from build123d import *

# Parameters (mm, degrees)
SKETCH1_W           = 56
SKETCH1_H           = 101
SKETCH1_R           = 1.65
BOSS_EXTRUDE1_DEPTH = 2
SKETCH3_W           = 56
SKETCH3_H           = 101
SKETCH3_W_2         = 50
SKETCH3_H_2         = 95
BOSS_EXTRUDE2_DEPTH = 15
SKETCH5_W           = 7
SKETCH5_H           = 72
CUT_EXTRUDE2_DEPTH  = 60.659450215


with BuildPart() as part:
    # Sketch1 → Boss-Extrude1 (new body)
    with BuildSketch(Plane(origin=(0, 0, 0), x_dir=(1, 0, 0), z_dir=(0, 1, 0))):
        Rectangle(SKETCH1_W, SKETCH1_H)
        with Locations(Location((-16.5, 40, 0), (0, 0, 270))):
            Circle(SKETCH1_R, mode=Mode.SUBTRACT)
        with Locations(Location((16.5, 40, 0), (0, 0, 270))):
            Circle(SKETCH1_R, mode=Mode.SUBTRACT)
        with Locations(Location((-16.5, -40, 0), (0, 0, 270))):
            Circle(SKETCH1_R, mode=Mode.SUBTRACT)
        with Locations(Location((16.5, -40, 0), (0, 0, 270))):
            Circle(SKETCH1_R, mode=Mode.SUBTRACT)
        Polygon((-12.964466094, -40), (12.964466094, -40), (16.5, -36.464466094), (16.5, 36.464466094), (12.964466094, 40), (-12.964466094, 40), (-16.5, 36.464466094), (-16.5, -36.464466094), align=None, mode=Mode.SUBTRACT)
    extrude(amount=BOSS_EXTRUDE1_DEPTH)

    # Sketch3 → Boss-Extrude2 (add)
    with BuildSketch(Plane(origin=(0, 2, 0), x_dir=(1, 0, 0), z_dir=(0, 1, 0))):
        Rectangle(SKETCH3_W, SKETCH3_H)
        Rectangle(SKETCH3_W_2, SKETCH3_H_2, mode=Mode.SUBTRACT)
    extrude(amount=BOSS_EXTRUDE2_DEPTH)

    # Sketch5 → Cut-Extrude2 (cut, through all)
    with BuildSketch(Plane(origin=(0, 2, 0), x_dir=(1, 0, 0), z_dir=(0, 1, 0))):
        with Locations((-20, 0)):
            Rectangle(SKETCH5_W, SKETCH5_H)
    extrude(amount=-CUT_EXTRUDE2_DEPTH, mode=Mode.SUBTRACT)


solid = part.part
Can you work these out from the model? Positions are in its coordinate system, mm. A direction names the side the tool comes from. Give positions to 0.01 mm unless a question says otherwise; leave off trailing zeros. Write each loop counter-clockwise with the first axis right and the second up, starting at its lowest first coordinate (ties: lowest second). Pieces come first, ordered by that corner, then holes. Notation, with made-up numbers: (-3.5, -37) -> (17.5, -37) arc R14 ccw to (17.5, -11) -> close; hole circle Ø11 at (79, 48.25). An arc over 180 degrees is marked (long way). Answer as a JSON object with one key per item and string values. Group by question number.
Item 1: Please list where these lines run through material, in increasing order: line 1 (Z direction, x = 11, y = 10.75); line 2 (X direction, y = 6.75, z = 18); line 3 (Y direction, x = -14.5, z = -40.5). Write a range as [from, to].
Item 2: For faces 4 (the face through (-20, 1, -36)), 5 (the face through (-25, 9, 1)), 6 (the face through (18, 0, -1)), which set-ups out of +Z, -Z, +X, -X, +Y, -Y let a thin tool reach every point of the face, with its end or its side?
Item 3: We'd pull the mould along X, two halves only. Please class faces 1 (the face through (-23.5, 1, 1)), 2 (the face through (28, 8, 1)), 3 (the face through (-27, 17, 4)): +X half, -X half, draft (parallel to the pull), parting line (faces both ways), or undercut.
Item 4: Suppose I cut it at C-C (y = 5.25). Please give me the cut outline in (x, z).
Item 5: Suppose I cut it at A-A (x = -8). Please give me the cut outline in (y, z), plus the area to 3 significant figures.
Item 6: Suppose I cut it at B-B (z = 9). Please give me the cut outline in (x, y), plus the area to 3 significant figures.
Item 7: Suppose I cut it at D-D (x = 24). Please give me the cut outline in (y, z), plus the area to 3 significant figures.
Findings:
{
 "1": {"line 1": "z = [-50.5, -47.5], [47.5, 50.5]", "line 2": "x = [-28, -25], [25, 28]", "line 3": "y = [0, 2]"},
 "2": {"face 4": "+Y, -Y", "face 5": "+Y", "face 6": "+Z, -Z, +X, -X, -Y"},
 "3": {"face 1": "undercut", "face 2": "+X half", "face 3": "draft"},
 "4": {"outline": "(-28, -50.5) -> (28, -50.5) -> (28, 50.5) -> (-28, 50.5) -> close; hole (-25, -47.5) -> (25, -47.5) -> (25, 47.5) -> (-25, 47.5) -> close"},
 "5": {"outline": "(0, -50.5) -> (17, -50.5) -> (17, -47.5) -> (2, -47.5) -> (2, -40) -> (0, -40) -> close; (0, 40) -> (2, 40) -> (2, 47.5) -> (17, 47.5) -> (17, 50.5) -> (0, 50.5) -> close", "area": "132 mm²"},
 "6": {"outline": "(-28, 0) -> (-23.5, 0) -> (-23.5, 2) -> (-25, 2) -> (-25, 17) -> (-28, 17) -> close; (16.5, 0) -> (28, 0) -> (28, 17) -> (25, 17) -> (25, 2) -> (16.5, 2) -> close", "area": "122 mm²"},
 "7": {"outline": "(0, -50.5) -> (17, -50.5) -> (17, -47.5) -> (2, -47.5) -> (2, 47.5) -> (17, 47.5) -> (17, 50.5) -> (0, 50.5) -> close", "area": "292 mm²"}
}
